from build123d import *

# Parameters (mm, degrees)
SKETCH1_W           = 150
SKETCH1_H           = 104
BOSS_EXTRUDE1_DEPTH = 92
SKETCH2_R           = 42
BOSS_EXTRUDE2_DEPTH = 44
FILLET1_R           = 3
FILLET2_R           = 3
SKETCH5_R           = 9.5
BOSS_EXTRUDE3_DEPTH = 8
FILLET3_R           = 1
SKETCH6_R           = 32.5
CUT_EXTRUDE1_DEPTH  = 5


with BuildPart() as part:
    # Sketch1 → Boss-Extrude1 (new body)
    with BuildSketch(Plane.XY):
        with Locations((75, 52)):
            Rectangle(SKETCH1_W, SKETCH1_H)
    extrude(amount=-BOSS_EXTRUDE1_DEPTH)

    # Sketch2 → Boss-Extrude2 (add)
    with BuildSketch(Plane.XY):
        with Locations((101, 54)):
            Circle(SKETCH2_R)
    extrude(amount=BOSS_EXTRUDE2_DEPTH)

    # Fillet1
    fillet1_edges = [part.edges().sort_by_distance(p)[0] for p in [
        (150, 52, -92),
        (75, 104, -92),
        (0, 52, -92),
        (75, 104, 0),
        (150, 52, 0),
        (75, 0, 0),
        (0, 52, 0),
        (0, 104, -46),
        (150, 104, -46),
        (150, 0, -46),
        (0, 0, -46),
        (75, 0, -92),
    ]]
    fillet(fillet1_edges, radius=FILLET1_R)

    # Fillet2
    fillet2_edges = [part.edges().sort_by_distance(p)[0] for p in [
        (59, 54, 0),
    ]]
    fillet(fillet2_edges, radius=FILLET2_R)

    # Sketch5 → Boss-Extrude3 (add)
    with BuildSketch(Plane(origin=(0, 104, 0), x_dir=(1, 0, 0), z_dir=(0, 1, 0))):
        with Locations(Location((23, 23, 0), (0, 0, 270))):
            Circle(SKETCH5_R)
    extrude(amount=BOSS_EXTRUDE3_DEPTH)

    # Fillet3
    fillet3_edges = [part.edges().sort_by_distance(p)[0] for p in [
        (23, 112, -32.5),
    ]]
    fillet(fillet3_edges, radius=FILLET3_R)

    # Sketch6 → Cut-Extrude1 (cut)
    with BuildSketch(Plane.XY.offset(44)):
        with Locations((101, 54)):
            Circle(SKETCH6_R)
    extrude(amount=-CUT_EXTRUDE1_DEPTH, mode=Mode.SUBTRACT)


solid = part.part
Read the model definition and answer for the solid it produces. Units are mm, in the model's axes. A direction names the side the tool comes from. Coordinates: 2 decimals unless noted, no trailing zeros. Loops run counter-clockwise (first coordinate to the right, second up) from the corner with the lowest first, then second, coordinate; pieces in that order, holes last.
Q1. The part is cut by section C-C on z = -70.5. Write down the section's boundary in (x, y).
Q2. The part is cut by section D-D on z = -23. Write down the section's boundary in (x, y), and give its area (3 significant figures).
Q3. Which of the six approach directions +Z, -Z, +X, -X, +Y, -Y give full straight-line access (tool end or side, diameter ignored) to faces 4 (the face through (67.67, 28.444, 23.213)), 5 (the face through (0, 51, -45))?
Q4. The mould has two halves that part along X. Classify faces 1 (the face through (68.53, 55.43, 41.54)), 2 (the face through (13.726, 107.451, -25.059)), 3 (the face through (123, 29, 44)): +X half, -X half, draft (parallel to the pull), parting line (faces both ways), or undercut.
Q5. Each of these flat-tipped pins is pushed along its axis until it touches: pin 1 Ø10 at (y, z) = (67, 20.5) entering from -X; pin 2 Ø6 at (x, z) = (131.5, 17) entering from -Y; pin 3 Ø6 at (x, y) = (111.5, 71.5) entering from +Z. Where does it stop, or does it pass through?
Q6. Consider probe 1 along Z at (x, y) = (99, 30); probe 2 along Y at (x, z) = (101, 41); probe 3 along Z at (x, y) = (61, 16.5). Determine where each line is inside the solid, lowest interval first.
Q7. The part is cut by section A-A on x = 23. Write down the section's boundary in (y, z), and give its area (3 significant figures).
Q8. The part is cut by section B-B on y = 54. Write down the section's boundary in (x, z).
Results below:
1. outline: (0, 3) arc R3 ccw to (3, 0) - (147, 0) arc R3 ccw to (150, 3) - (150, 101) arc R3 ccw to (147, 104) - (3, 104) arc R3 ccw to (0, 101) - close
2. outline: (0, 3) arc R3 ccw to (3, 0) - (147, 0) arc R3 ccw to (150, 3) - (150, 101) arc R3 ccw to (147, 104) - (32.5, 104) - (32.5, 111) arc R1 ccw to (31.5, 112) - (14.5, 112) arc R1 ccw to (13.5, 111) - (13.5, 104) - (3, 104) arc R3 ccw to (0, 101) - close
2. area: 15,700 mm2
3. face 4: +Z
3. face 5: +Z, -Z, -X, +Y, -Y
4. face 1: undercut
4. face 2: parting line
4. face 3: draft
5. pin 1: stops at x = 59.77
5. pin 2: stops at y = 22.25
5. pin 3: stops at z = 39
6. probe 1: z = -92 to 39
6. probe 2: y = 12 to 21.5, 86.5 to 96
6. probe 3: z = -92 to 0
7. outline: (0, -89) arc R3 ccw to (3, -92) - (101, -92) arc R3 ccw to (104, -89) - (104, -32.5) - (111, -32.5) arc R1 ccw to (112, -31.5) - (112, -14.5) arc R1 ccw to (111, -13.5) - (104, -13.5) - (104, -3) arc R3 ccw to (101, 0) - (3, 0) arc R3 ccw to (0, -3) - close
7. area: 9,710 mm2
8. outline: (0, -89) arc R3 ccw to (3, -92) - (147, -92) arc R3 ccw to (150, -89) - (150, -3) arc R3 ccw to (147, 0) - (146, 0) arc R3 cw to (143, 3) - (143, 44) - (133.5, 44) - (133.5, 39) - (68.5, 39) - (68.5, 44) - (59, 44) - (59, 3) arc R3 cw to (56, 0) - (3, 0) arc R3 ccw to (0, -3) - close
